Drawing for the job (mm, zero at the part's lowest x, y, z). Round coordinates to 2 decimals unless told otherwise and drop trailing zeros. Loops run counter-clockwise (first coordinate to the right, second up) from the corner with the lowest first, then second, coordinate; pieces in that order, holes last. Notation, with made-up numbers: M 38,81.5 L 79,81.5 A21 cw 79,118.5 Z; hole C -22,30.5 d3. An arc over 180 degrees is marked long. Write each question's results on one line, items separated by ' | '.
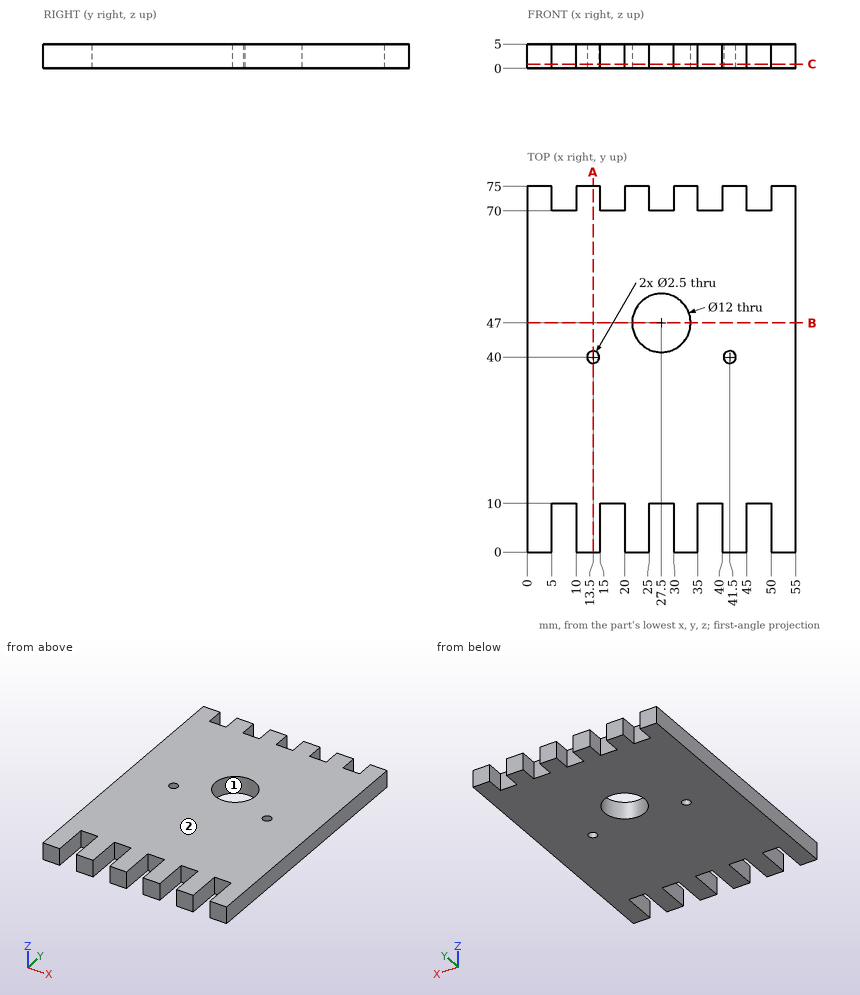
Item 1: Wall check: L1, parallel to X at y = 5.5, z = 1.1; L2, parallel to Y at x = 13.5, z = 2; L3, parallel to Y at x = 27.5, z = 2.1. Give the ranges that are in metal, low to high.
Filled sheet:
L1: 0 to 5, 10 to 15, 20 to 25, 30 to 35, 40 to 45, 50 to 55 | L2: 0 to 38.75, 41.25 to 75 | L3: 10 to 41, 53 to 70
Item 2: Band-saw the part on B-B on y = 47. Give the cut face in (x, z), and give its area (3 significant figures).
Filled sheet:
outline: M 0,0 L 21.5,0 L 21.5,5 L 0,5 Z; M 33.5,0 L 55,0 L 55,5 L 33.5,5 Z | area: 215 mm^2
Item 3: Band-saw the part on C-C on z = 0.85. Count the separate pieces of the cut face and the enclosed holes in it, and give its area (3 significant figures).
Filled sheet:
separate pieces: 1 | enclosed holes: 3 | area: 3,630 mm^2
Item 4: Band-saw the part on A-A on x = 13.5. Give the cut face in (y, z), and give its area (4 significant figures).
Filled sheet:
outline: M 0,0 L 38.75,0 L 38.75,5 L 0,5 Z; M 41.25,0 L 75,0 L 75,5 L 41.25,5 Z | area: 362.5 mm^2
Item 5: Two-plate mould, pull along X, no slides. Class the marked faces 1 and 2: +X half, -X half, draft (parallel to the pull), parting line (faces both ways), or undercut.
Filled sheet:
face 1: undercut | face 2: draft
Item 6: Drop flat-ended pins along their axis: P1, Ø1.5, axis at x = 47.5, z = 1.5, coming from the +Y side; P2, Ø1.5, axis at x = 28.5, z = 1.5, coming from the -Y side; P3, Ø7, axis at x = 27.5, y = 47, coming from the -Z side. Give the stop position or say it passes through.
Filled sheet:
P1: y = 70 | P2: y = 10 | P3: through
